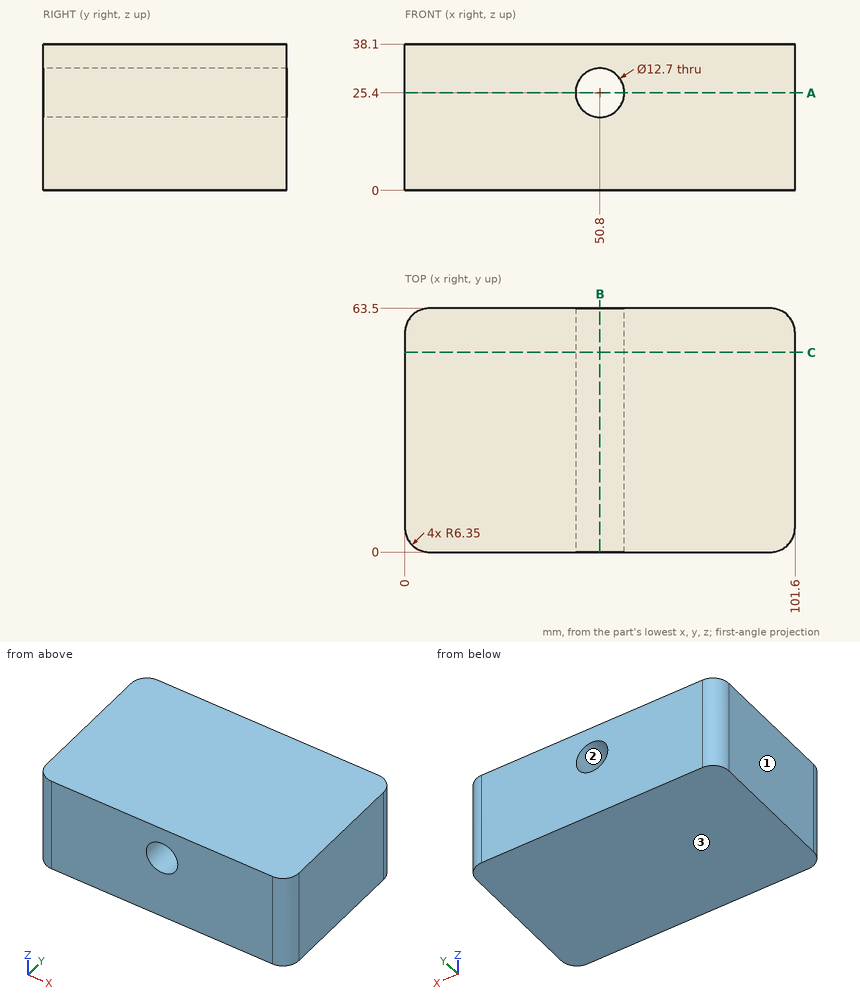
Answer from the drawing. Dimensions are ordinates in mm from the lowest x, y and z of the part. Give positions to 0.01 mm unless a question says otherwise; leave off trailing zeros. Write each loop counter-clockwise with the first axis right and the second up, starting at its lowest first coordinate (ties: lowest second). Pieces come first, ordered by that corner, then holes. Notation, with made-up numbers: (-24.5, 19.5) - (16.5, 19.5) arc R33 ccw to (16.5, 51.5) - close; hole circle Ø9 at (78, 52.5). An arc over 180 degrees is marked (long way). One line per item, written item: value. Start each with the question number.
1. For a pull along Z with two mould halves and no side action, classify the marked faces 1, 2 and 3 as +Z half, -Z half, draft (parallel to the pull), parting line (faces both ways), or undercut.
2. Find section B-B (x = 50.8). Write down the section's boundary in (y, z).
3. Consider probe 1 along X at (y, z) = (33, 25); probe 2 along Z at (x, y) = (49, 36); probe 3 along X at (y, z) = (34.5, 27.5). Determine where each line is inside the solid, lowest interval first.
4. Find section C-C (y = 52). Write down the section's boundary in (x, z), then the cut area to 3 significant figures.
5. Find section A-A (z = 25.4). Write down the section's boundary in (x, y).
6. Given pin 1 (2 mm diameter, centred on x = 87, y = 52, fed in from -Z); pin 2 (7.5 mm diameter, centred on x = 50.8, z = 25.4, fed in from -Y), each flat-ended and moving along its own axis, determine where each tip first touches the part or whether it passes through.
Geometry results:
1. face 1: draft
1. face 2: undercut
1. face 3: -Z half
2. outline: (0, 0) - (63.5, 0) - (63.5, 19.05) - (0, 19.05) - close; (0, 31.75) - (63.5, 31.75) - (63.5, 38.1) - (0, 38.1) - close
3. probe 1: 0 to 44.46, 57.14 to 101.6
3. probe 2: 0 to 19.31, 31.49 to 38.1
3. probe 3: 0 to 44.81, 56.79 to 101.6
4. outline: (0, 0) - (101.6, 0) - (101.6, 38.1) - (0, 38.1) - close; hole circle Ø12.7 at (50.8, 25.4)
4. area: 3,740 mm2
5. outline: (0, 6.35) arc R6.35 ccw to (6.35, 0) - (44.45, 0) - (44.45, 63.5) - (6.35, 63.5) arc R6.35 ccw to (0, 57.15) - close; (57.15, 0) - (95.25, 0) arc R6.35 ccw to (101.6, 6.35) - (101.6, 57.15) arc R6.35 ccw to (95.25, 63.5) - (57.15, 63.5) - close
6. pin 1: z = 0
6. pin 2: through
